Source: three-view drawing plus pictorial views. Frame: mm from the lowest corner of the part. A direction names the side the tool comes from. Give positions to 0.01 mm unless a question says otherwise; leave off trailing zeros. Order: outer loops, then holes, each group sorted by start corner. A loop starts at its lowest first (then second) coordinate and runs counter-clockwise, first axis right, second up. Notation, with made-up numbers: (77.5, -19) -> (104.5, -19) arc R27 ccw to (104.5, -3) -> close; hole circle Ø9 at (-12.75, -28). An arc over 180 degrees is marked (long way). Answer in a Markdown table with one row per item. Add a question column.
Q1. Set-up query: the marked faces 1, 2 and 3. Return all of +Z, -Z, +X, -X, +Y, -Y with unobstructed straight access to the full face (end or side cutting, diameter ignored); none if empty.
Q2. Line query: line 1 along X through (y, z) = (6, 3); line 2 along X through (y, z) = (24, 18.75); line 3 along Y through (x, z) = (18, 6.25). Output: solid intervals per line, ascending. Write a range as from..to.
Q3. Cut plane D-D on y = 44. Return the cut outline in (x, z), and give its area (3 significant figures).
Q4. Cut plane C-C on x = 15. Return the cut outline in (y, z), and give its area (3 significant figures).
Q5. Cut plane A-A on z = 15. Return the cut outline in (x, y).
Q6. Contact query for flat-ended pins moving along their axis: P1, Ø14.5, axis at y = 30, z = 12.5, coming from the +X side; P2, Ø5, axis at x = 10.5, y = 21, coming from the +Z side; P3, Ø4, axis at x = 15, z = 27, coming from the +Y side; P4, Ø2.5, axis at x = 15, z = 3, coming from the -Y side. Output: stop coordinate, or through.
Q7. Pull-direction query (Y, two-part tool) for the marked faces 4, 5 and 6; classes: +Y half, -Y half, draft (parallel to the pull), parting line (faces both ways), or undercut.
Q8. Cut plane B-B on y = 3. Return the cut outline in (x, z).
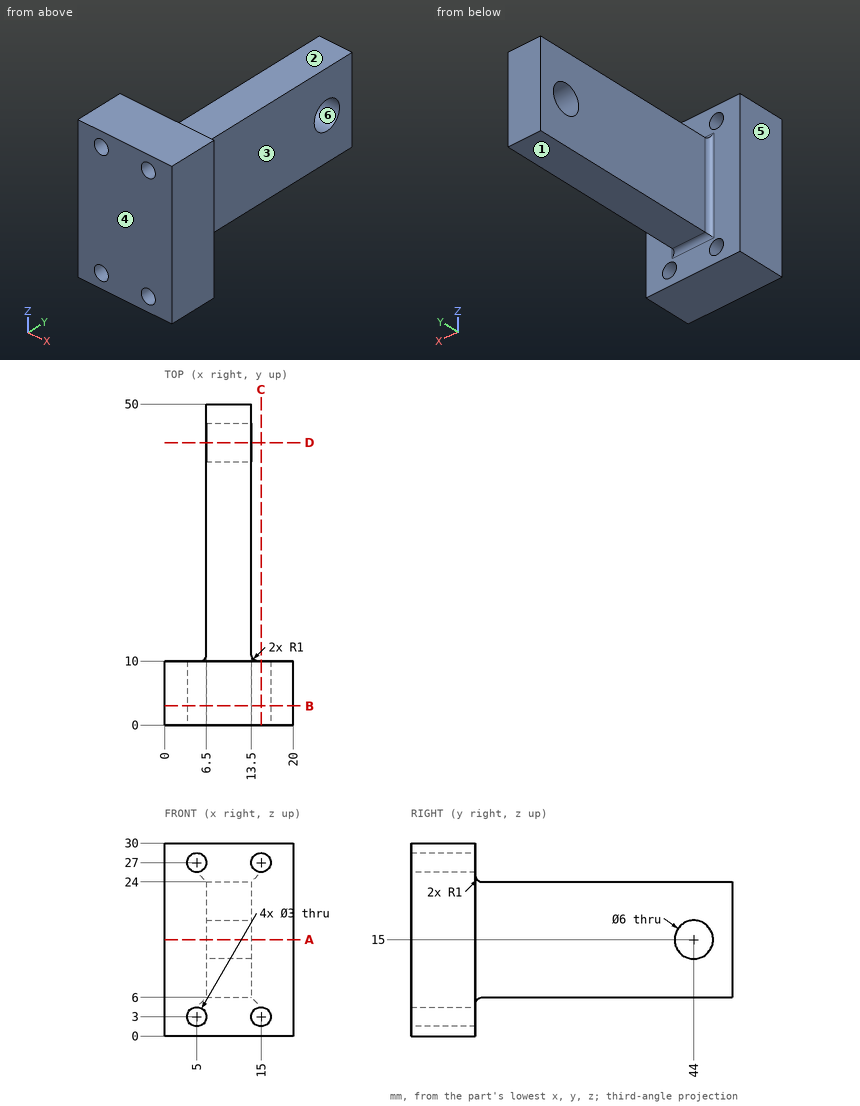
Completed:
| question | item | result |
|---|---|---|
| 1 | face 1 | -Z, +X, -X, +Y |
| 1 | face 2 | +Z, +X, -X, +Y |
| 1 | face 3 | +Z, -Z, +X, +Y |
| 2 | line 1 | x = 0..3.5, 6.5..13.5, 16.5..20 |
| 2 | line 2 | x = 6.5..13.5 |
| 2 | line 3 | y = 0..10 |
| 3 | outline | (6.5, 6) -> (13.5, 6) -> (13.5, 12) -> (6.5, 12) -> close; (6.5, 18) -> (13.5, 18) -> (13.5, 24) -> (6.5, 24) -> close |
| 3 | area | 84.0 mm² |
| 4 | outline | (0, 0) -> (10, 0) -> (10, 1.5) -> (0, 1.5) -> close; (0, 4.5) -> (10, 4.5) -> (10, 25.5) -> (0, 25.5) -> close; (0, 28.5) -> (10, 28.5) -> (10, 30) -> (0, 30) -> close |
| 4 | area | 240 mm² |
| 5 | outline | (0, 0) -> (20, 0) -> (20, 10) -> (14.5, 10) arc R1 cw to (13.5, 11) -> (13.5, 41) -> (6.5, 41) -> (6.5, 11) arc R1 cw to (5.5, 10) -> (0, 10) -> close; (6.5, 47) -> (13.5, 47) -> (13.5, 50) -> (6.5, 50) -> close |
| 6 | P1 | stops at x = 13.5 |
| 6 | P2 | stops at z = 24 |
| 6 | P3 | stops at y = 10 |
| 6 | P4 | passes through |
| 7 | face 4 | -Y half |
| 7 | face 5 | draft |
| 7 | face 6 | undercut |
| 8 | outline | (0, 0) -> (20, 0) -> (20, 30) -> (0, 30) -> close; hole circle Ø3 at (5, 3); hole circle Ø3 at (5, 27); hole circle Ø3 at (15, 3); hole circle Ø3 at (15, 27) |
